Can you work these out from the drawing? Everything is in mm from the part's minimum corner. A direction names the side the tool comes from. Coordinates: 2 decimals unless noted, no trailing zeros. Write each loop counter-clockwise with the first axis right and the second up, starting at its lowest first coordinate (ties: lowest second). Pieces come first, ordered by that corner, then holes. Notation, with made-up numbers: (86.25, 30.25) -> (123.25, 30.25) arc R26 cw to (123.25, 50.25) -> close; hole circle Ø2 at (45.5, 53.5). An arc over 180 degrees is marked (long way). Use a Markdown table: item, result. Add a question column.
Item 1: On a 3-axis mill with a long thin cutter (end or side, diameter ignored), from which of +Z, -Z, +X, -X, +Y, -Y can I reach the whole of each face in a straight line? I mean the marked faces 1 and 2. Say none if no direction works.
Item 2: Imagine slicing it at D-D, the plane x = 8.6. Write out the boundary of the cut face in (y, z), and give its area (3 significant figures).
Item 3: Imagine slicing it at B-B, the plane z = 7.75. Write out the boundary of the cut face in (x, y).
Item 4: Imagine slicing it at C-C, the plane x = 29. Write out the boundary of the cut face in (y, z).
Item 5: Imagine slicing it at A-A, the plane x = 86.8. Write out the boundary of the cut face in (y, z), and give its area (3 significant figures).
Item 6: Will these pins go through, and if not, where does the flat tip stop? pin 1 Ø6 at (x, z) = (43.5, 10.5) entering from +Y; pin 2 Ø4 at (x, y) = (8.6, 97.6) entering from +Z; pin 3 Ø1.5 at (y, z) = (48.5, 12.5) entering from +X.
Item 7: If I drill on line 1 along Y through (x, z) = (36.8, 0.7); line 2 along Y through (x, z) = (8.6, 0.35); line 3 along Y through (x, z) = (77, 5.5), over which ranges is the centre line in solid material (lowest first)? Write a range as from..to.
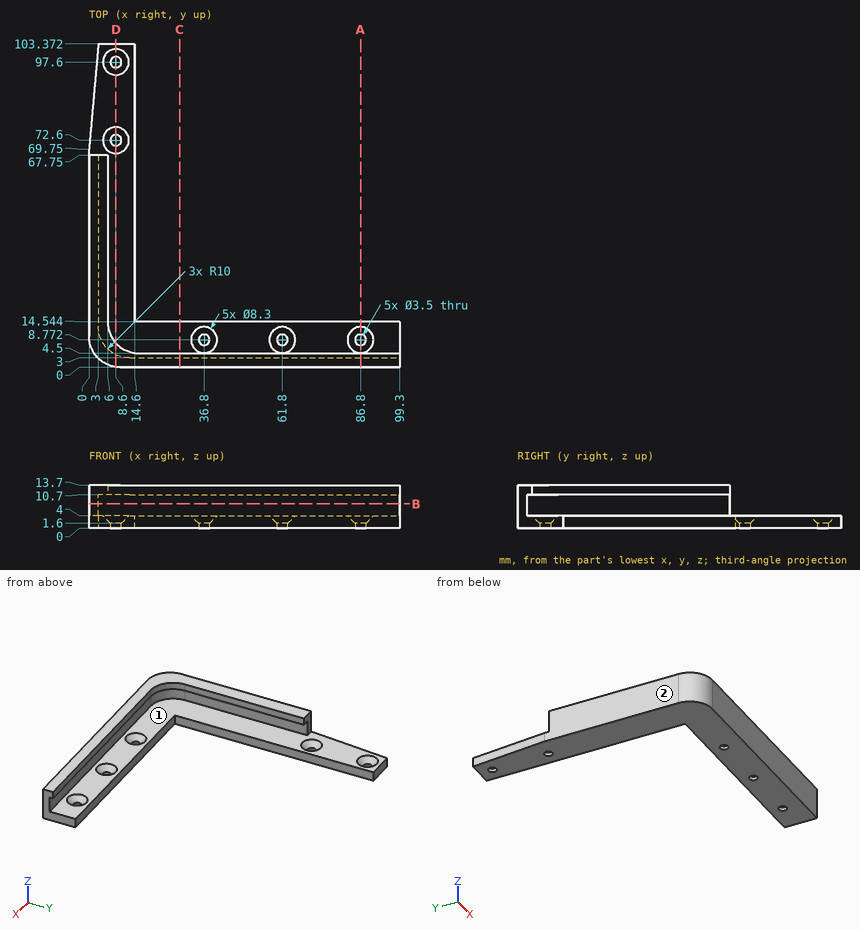
Ans:
| question | item | result |
|---|---|---|
| 1 | face 1 | +X, +Y |
| 1 | face 2 | +Z, -Z, -X, +Y, -Y |
| 2 | outline | (0.1, 0) -> (70.85, 0) -> (70.85, 1.6) -> (68.45, 4) -> (4.02, 4) -> (4.02, 10.7) -> (7.77, 10.7) -> (7.77, 13.7) -> (0.1, 13.7) -> close; (74.35, 0) -> (95.85, 0) -> (95.85, 1.6) -> (93.45, 4) -> (76.75, 4) -> (74.35, 1.6) -> close; (99.35, 0) -> (103.37, 0) -> (103.37, 4) -> (101.75, 4) -> (99.35, 1.6) -> close |
| 2 | area | 423 mm^2 |
| 3 | outline | (0, 10) arc R10 ccw to (10, 0) -> (99.3, 0) -> (99.3, 3) -> (13, 3) arc R10 cw to (3, 13) -> (3, 67.75) -> (0, 67.75) -> close |
| 4 | outline | (0, 0) -> (14.54, 0) -> (14.54, 4) -> (3, 4) -> (3, 10.7) -> (4.5, 10.7) -> (4.5, 13.7) -> (0, 13.7) -> close |
| 5 | outline | (0, 0) -> (7.02, 0) -> (7.02, 1.6) -> (4.62, 4) -> (3, 4) -> (3, 10.7) -> (4.5, 10.7) -> (4.5, 13.7) -> (0, 13.7) -> close; (10.52, 0) -> (14.54, 0) -> (14.54, 4) -> (12.92, 4) -> (10.52, 1.6) -> close |
| 5 | area | 72.0 mm^2 |
| 6 | pin 1 | stops at y = 4.5 |
| 6 | pin 2 | stops at z = 1.85 |
| 6 | pin 3 | stops at x = 6 |
| 7 | line 1 | y = 0..7.02, 10.52..14.54 |
| 7 | line 2 | y = 0.1..70.85, 74.35..95.85, 99.35..103.37 |
| 7 | line 3 | y = 0..3 |
